Design review of the part built by this model. Coordinates are the model's own, in mm. Coordinates: 2 decimals unless noted, no trailing zeros. One line per item, written item: value.
Autodesk Inventor part; units mm, degrees
ref_plane "YZ Plane" through (0, 0, 0) normal (1, 0, 0) x (0, 1, 0)
ref_plane "XZ Plane" through (0, 0, 0) normal (0, 1, 0) x (-1, 0, 0)
ref_plane "XY Plane" through (0, 0, 0) normal (0, 0, 1) x (1, 0, 0)
sketch "Sketch1" plane through (0, 0, 0) normal (0, 1, 0) x (-1, 0, 0)
  line L0 (114.3, 114.3) -> (-114.3, 114.3)
  line L1 (-114.3, 114.3) -> (-114.3, -114.3)
  line L2 (-114.3, -114.3) -> (114.3, -114.3)
  line L3 (114.3, -114.3) -> (114.3, 114.3)
  point P0 (0, 0)
  dimension "d0" = 228.6
  dimension "d1" = 228.6
extrude "Extrusion1" add sketch "Sketch1" along normal blind 6.35
sketch "Sketch2" plane through (114.3, 0, 114.3) normal (1, 0, 0) x (0, 0, -1)
  line L0 (0, 3.175) -> (38.1, 3.175)
  line L1 (38.1, 3.175) -> (76.2, 3.175)
  line L2 (76.2, 3.175) -> (114.3, 3.175)
  line L3 (114.3, 3.175) -> (152.4, 3.175)
  line L4 (152.4, 3.175) -> (190.5, 3.175)
  line L5 (190.5, 3.175) -> (228.6, 3.175)
  line L6 (228.6, 0) -> (228.6, 3.175)
  point P0 (114.3, 0)
  point P1 (0, 0)
  dimension "d4" = 38.1
  dimension "d5" = 38.1
  dimension "d6" = 38.1
  dimension "d7" = 38.1
  dimension "d8" = 38.1
  dimension "d85" = 3.175
hole "Hole1" at (114.3, 3.175, 76.2) at (114.3, 3.175, 38.1) at (114.3, 3.175, 0) at (114.3, 3.175, -38.1) at (114.3, 3.175, -76.2) direction (-1, 0, 0) diameter 2.1565 depth 8.8646
sketch "Sketch3" plane through (114.3, 0, -114.3) normal (0, 0, -1) x (-1, 0, 0)
  line L0 (0, 0) -> (0, 3.175)
  line L1 (0, 3.175) -> (38.1, 3.175)
  line L2 (38.1, 3.175) -> (76.2, 3.175)
  line L3 (76.2, 3.175) -> (114.3, 3.175)
  line L4 (114.3, 3.175) -> (152.4, 3.175)
  line L5 (152.4, 3.175) -> (190.5, 3.175)
  line L6 (190.5, 3.175) -> (228.6, 3.175)
  line L7 (228.6, 0) -> (228.6, 6.35)
  point P0 (114.3, 0)
  dimension "d16" = 38.1
  dimension "d17" = 38.1
  dimension "d18" = 38.1
  dimension "d19" = 38.1
  dimension "d20" = 38.1
  dimension "d83" = 3.175
hole "Hole2" at (76.2, 3.175, -114.3) at (38.1, 3.175, -114.3) at (0, 3.175, -114.3) at (-38.1, 3.175, -114.3) at (-76.2, 3.175, -114.3) direction (0, 0, 1) diameter 2.1565 depth 8.8646
sketch "Sketch4" plane through (-114.3, 0, -114.3) normal (-1, 0, 0) x (0, 0, 1)
  line L0 (0, 3.175) -> (38.1, 3.175)
  line L1 (38.1, 3.175) -> (76.2, 3.175)
  line L2 (76.2, 3.175) -> (114.3, 3.175)
  line L3 (114.3, 3.175) -> (152.4, 3.175)
  line L4 (152.4, 3.175) -> (190.5, 3.175)
  line L5 (0, 3.175) -> (0, 0)
  point P0 (114.3, 0)
  dimension "d28" = 38.1
  dimension "d29" = 38.1
  dimension "d30" = 38.1
  dimension "d31" = 38.1
  dimension "d32" = 38.1
  dimension "d86" = 3.175
hole "Hole3" at (-114.3, 3.175, -76.2) at (-114.3, 3.175, -38.1) at (-114.3, 3.175, 0) at (-114.3, 3.175, 38.1) at (-114.3, 3.175, 76.2) direction (1, 0, 0) diameter 2.1565 depth 8.8646
sketch "Sketch5" plane through (-114.3, 0, 114.3) normal (0, 0, 1) x (1, 0, 0)
  line L0 (0, 0) -> (0, 3.175)
  line L1 (0, 0) -> (0, 6.35)
  line L2 (0, 3.175) -> (38.1, 3.175)
  line L3 (0, 3.175) -> (38.1, 3.175) construction
  line L4 (38.1, 3.175) -> (76.2, 3.175)
  line L5 (76.2, 3.175) -> (114.3, 3.175)
  line L6 (114.3, 3.175) -> (152.4, 3.175)
  line L7 (152.4, 3.175) -> (190.5, 3.175)
  point P0 (114.3, 0)
  dimension "d40" = 3.175
  dimension "d41" = 38.1
  dimension "d42" = 0
  dimension "d43" = 38.1
  dimension "d44" = 38.1
  dimension "d45" = 38.1
  dimension "d46" = 38.1
hole "Hole4" at (-76.2, 3.175, 114.3) at (-38.1, 3.175, 114.3) at (0, 3.175, 114.3) at (38.1, 3.175, 114.3) at (76.2, 3.175, 114.3) direction (0, 0, -1) diameter 2.1565 depth 8.8646
sketch "Sketch6" plane through (0, 0, 0) normal (0, 1, 0) x (1, 0, 0)
  line L0 (-114.3, -114.3) -> (114.3, -114.3)
  line L1 (-114.3, -114.3) -> (-12.7, -114.3)
  line L2 (-12.7, -114.3) -> (-12.7, -63.5)
  line L3 (-12.7, -63.5) -> (-12.7, -23.622)
  line L4 (114.3, -114.3) -> (57.15, -114.3)
  line L5 (57.15, -114.3) -> (57.15, -63.5)
  line L6 (57.15, -63.5) -> (57.15, -23.622)
  line L7 (-114.3, 114.3) -> (-114.3, -114.3)
  line L8 (-114.3, 114.3) -> (-114.3, 57.15)
  line L9 (-114.3, 57.15) -> (38.1, 57.15)
  line L10 (38.1, 57.15) -> (77.978, 57.15)
  point P0 (0, 0)
  dimension "d54" = 101.6
  dimension "d55" = 50.8
  dimension "d56" = 39.878
  dimension "d57" = 57.15
  dimension "d58" = 57.15
  dimension "d59" = 152.4
  dimension "d60" = 39.878
hole "Hole5" at (77.978, 0, -57.15) at (38.1, 0, -57.15) at (-12.7, 0, 63.5) at (-12.7, 0, 23.622) at (57.15, 0, 23.622) at (57.15, 0, 63.5) direction (0, 1, 0) diameter 3.556 end through all countersink diameter 9.525 countersink angle 82
sketch "Sketch8" plane through (0, 6.35, 0) normal (0, 1, 0) x (1, 0, 0)
  circle A0 centre (57.15, -23.622) radius 1.778
  circle A1 centre (-12.7, -63.5) radius 1.778
  circle A2 centre (77.978, 57.15) radius 1.778
  circle A3 centre (38.1, 57.15) radius 1.778
  circle A4 centre (-12.7, -23.622) radius 1.778
  circle A5 centre (57.15, -63.5) radius 1.778
  line L0 (114.3, -114.3) -> (114.3, 114.3)
  line L1 (114.3, 114.3) -> (-114.3, 114.3)
  line L2 (-114.3, 114.3) -> (-114.3, -114.3)
  line L3 (-114.3, -114.3) -> (114.3, -114.3)
  point P0 (0, 0)
properties part number "sheetmetalbottom2.0"
(1) Insertion check: pin 1 (1.1 mm diameter, centred on x = 76.5, y = 3, fed in from -Z); pin 2 (0.6 mm diameter, centred on y = 2.5, z = -0.5, fed in from -X); pin 3 (1.1 mm diameter, centred on x = 76, y = 3.5, fed in from +Z); pin 4 (1.7 mm diameter, centred on y = 3.175, z = 0, fed in from +X). Each pin has a flat end and moves straight along its axis. Give the tip position at first contact, or say it passes through.
Reply:
pin 1: stops at z = -105.44
pin 2: stops at x = -114.3
pin 3: stops at z = 105.44
pin 4: stops at x = 105.44
(2) Mouldability with a two-part tool opening along Z and no side actions: class faces 1 (the flat face through (2, 3, -114.3)), 2 (the conical face through (36.182, 3.219, -56.724)), 3 (the flat face through (114.3, 3, 2)) as released by +Z, released by -Z, zero draft, split by the parting line, or undercut.
Reply:
face 1: released by -Z
face 2: undercut
face 3: zero draft
(3) To check wall thickness, follow line 1 along Y through (x, z) = (0, -110.5). State the ranges of the line that lie inside material, in increasing order. Write a range as [from, to].
Reply:
line 1: y = [0, 2.1], [4.25, 6.35]
